```python
from build123d import *

# Parameters (mm, degrees)
F0_W            = 200
F0_H            = 150
F1_DEPTH        = 80
F13_D           = 9
F13_CSINK_D     = 18
F13_CSINK_ANGLE = 90
F2_R            = 16.4559911856
F3_DEPTH        = 60
F4_DEPTH        = 25
F14_R           = 5
F5_R            = 5
F11_DEPTH       = 22


# Not quite as in the source:
# - a pattern or mirror of a feature is missing from the dataset's text; its kind, count and spacing are read off the source's solid


with BuildPart() as f1:
    # F0 (on Top) → F1 (new body)
    with BuildSketch(Plane.XY):
        Rectangle(F0_W, F0_H)
    extrude(amount=F1_DEPTH)

    # F13 (through all)
    with Locations(Plane.XY.offset(80)):
        with Locations((-60, 35), (-60, -45), (60, 35), (60, -45)):
            CounterSinkHole(F13_D / 2, F13_CSINK_D / 2, counter_sink_angle=F13_CSINK_ANGLE)

    # F2 (on face) → F4 (join)
    with BuildSketch(Plane.YZ.offset(100)):
        with Locations((-21.9944119453, 55.6955486536)):
            Circle(F2_R)
    extrude(amount=F4_DEPTH)

    # F14
    f14_edges = [f1.edges().sort_by_distance(p)[0] for p in [
        (100, -38.450403, 55.695549),
        (125, -38.450403, 55.695549),
    ]]
    fillet(f14_edges, radius=F14_R)

    # F7 (on face) → F15 (revolve)
    with BuildSketch(Plane.XZ.offset(75)):
        Polygon((8, 58.6291704433), (33, 15.327900254), (58, 58.6291704433), align=None)
    revolve(axis=Axis((0, -75, 40), (0, 0, -1)))

    # F10 (on face) → F11 (join)
    with BuildSketch(Plane(origin=(-100, 0, 0), x_dir=(0, -1, 0), z_dir=(-1, 0, 0))):
        Polygon((-20, 65), (-65, 65), (-65, 10), (-20, 10), (-20, 30), (-42.5, 30), align=None)
    f11 = extrude(amount=F11_DEPTH)

    # F11_copies: F11 across plane
    add(f11.mirror(Plane(origin=(0, 0, 0), x_dir=(0, 0, -1), z_dir=(0, -1, 0))))


with BuildPart() as f3:
    # F2 (on face) → F3 (new body)
    with BuildSketch(Plane.YZ.offset(100)):
        with Locations((78.0055880547, 135.6955486536)):
            Circle(F2_R)
    extrude(amount=F3_DEPTH)

    # F5
    f5_edges = [f3.edges().sort_by_distance(p)[0] for p in [
        (160, 61.549597, 135.695549),
        (100, 61.549597, 135.695549),
    ]]
    fillet(f5_edges, radius=F5_R)


with BuildPart() as f6_1:
    # F6: instance of F3
    add(f3.part.mirror(Plane.YZ))


solid = f1.part
```
Part model, mm, in its own coordinate system. A direction names the side the tool comes from. Round coordinates to 2 decimals unless told otherwise and drop trailing zeros. Write each loop counter-clockwise with the first axis right and the second up, starting at its lowest first coordinate (ties: lowest second). Pieces come first, ordered by that corner, then holes. Notation, with made-up numbers: M 55,-5 L 89,-5 A9 cw 89,0 Z; hole C -4,44.25 d8. An arc over 180 degrees is marked long. One line per question, with ' | ' between items.
(1) 3-axis set-ups, long thin cutter, end or side, ignore diameter. For faces 1 (the face through (0.39, -92.89, 41.49)), 2 (the face through (-111, -31, 30)), 3 (the face through (-1, -98, 58.629)), 4 (the face through (-111, -43, 10)): which of +Z, -Z, +X, -X, +Y, -Y reach the whole face in a straight line?
Answer key:
face 1: -Z | face 2: -X | face 3: +Z, +X, -X, -Y | face 4: -Z, -X, +Y, -Y
(2) Saw through at A-A on y = 35. Write the cut outline in (x, z), then the cut area to 3 significant figures.
Answer key:
outline: M -122,10 L -100,10 L -100,0 L -64.5,0 L -64.5,75.5 L -69,80 L -100,80 L -100,65 L -122,65 L -122,41.67 L -100,41.67 L -100,30 L -122,30 Z; M -55.5,0 L 55.5,0 L 55.5,75.5 L 51,80 L -51,80 L -55.5,75.5 Z; M 64.5,0 L 100,0 L 100,80 L 69,80 L 64.5,75.5 Z | area: 15,500 mm^2
(3) Saw through at B-B on x = -87. Write the cut outline in (y, z), then the cut area to 3 significant figures.
Answer key:
outline: M -75,0 L 75,0 L 75,80 L -75,80 Z | area: 12,000 mm^2
(4) Two-plate mould, pull along X, no slides. Class faces 5 (the face through (-111, 65, 38)), 6 (the face through (-122, 48, 38)), 7 (the face through (64, -48, 76)): released by +X, released by -X, zero draft, split by the parting line, or undercut.
Answer key:
face 5: zero draft | face 6: released by -X | face 7: undercut
(5) Pin check, flat tips, straight feed: pin 1 (2 mm diameter, centred on x = -85.5, y = -41.5, fed in from -Z); pin 2 (4 mm diameter, centred on x = 7.5, z = 63, fed in from -Y); pin 3 (6 mm diameter, centred on x = -106.5, z = 15, fed in from -Y); pin 4 (10 mm diameter, centred on x = -114, z = 15.5, fed in from +Y). Stop position of each tip, or through.
Answer key:
pin 1: stops at z = 0 | pin 2: stops at y = -75 | pin 3: stops at y = -65 | pin 4: stops at y = 65
(6) Probe line 1 along X through (y, z) = (-45, 53); line 2 along Y through (x, z) = (-60, 46); line 3 along X through (y, z) = (-42.5, 6.5). List the from-to ranges inside material, lowest first.
Answer key:
line 1: x = -122 to -64.5, -55.5 to 55.5, 64.5 to 100 | line 2: y = -75 to -49.5, -40.5 to 30.5, 39.5 to 75 | line 3: x = -100 to -63.74, -56.26 to 56.26, 63.74 to 100
(7) Saw through at D-D on x = 61. Count the separate pieces of the cut face and the enclosed holes in it, then the cut area to 3 significant figures.
Answer key:
separate pieces: 3 | enclosed holes: 0 | area: 10,600 mm^2
(8) Saw through at C-C on y = -70.5. Write the cut outline in (x, z), then the cut area to 3 significant figures.
Answer key:
outline: M -100,0 L 100,0 L 100,80 L -100,80 Z | area: 16,000 mm^2
